from build123d import *

# Parameters (mm, degrees)
RESSALTO_EXTRUS_O1_DEPTH   = 5
CORTE_EXTRUS_O1_DEPTH      = 83.83115356
CORTE_EXTRUS_O1_DEPTH_BACK = 4
ESBO_O5_W                  = 35
ESBO_O5_H                  = 10
RESSALTO_EXTRUS_O2_DEPTH   = 5
FILETE1_R                  = 5
CORTE_EXTRUS_O2_DEPTH      = 83.83115356
CORTE_EXTRUS_O3_DEPTH      = 5
FILETE2_R                  = 2
ESBO_O10_W                 = 20
ESBO_O10_H                 = 50
CORTE_EXTRUS_O4_DEPTH      = 84.282651255


with BuildPart() as part:
    # Esboço1 → Ressalto-extrusão1 (new body)
    with BuildSketch(Plane.XY):
        Polygon((0, 0), (0, 70), (20, 70), (20, 20), (44, 20), (44, 0), align=None)
    extrude(amount=RESSALTO_EXTRUS_O1_DEPTH)

    # Esboço5 → Corte-extrusão1 (cut, two sides: drawn at the far end of the back side and taken through both)
    with BuildSketch(Plane.XY.offset(5).offset(-CORTE_EXTRUS_O1_DEPTH_BACK)):
        with Locations((26.5, 9)):
            Rectangle(ESBO_O5_W, ESBO_O5_H)
    extrude(amount=CORTE_EXTRUS_O1_DEPTH + CORTE_EXTRUS_O1_DEPTH_BACK, mode=Mode.SUBTRACT)

    # Esboço6 → Ressalto-extrusão2 (add)
    with BuildSketch(Plane.XY.offset(5)):
        Polygon((44, 20), (0, 20), (0, 0), (44, 0), (44, 4), (9, 4), (9, 14), (44, 14), align=None)
    extrude(amount=RESSALTO_EXTRUS_O2_DEPTH)

    # Filete1
    filete1_edges = [part.edges().sort_by_distance(p)[0] for p in [
        (10, 20, 5),
    ]]
    fillet(filete1_edges, radius=FILETE1_R - 0.0001)  # a hair under: the kernel refuses the full size

    # Esboço7 → Corte-extrusão2 (cut, through all)
    with BuildSketch(Plane.XY.offset(5)):
        with BuildLine():
            Line((12.75, 65), (12.75, 55))
            ThreePointArc((12.75, 55), (10, 52.25), (7.25, 55))
            Line((7.25, 55), (7.25, 65))
            ThreePointArc((7.25, 65), (10, 67.75), (12.75, 65))
        make_face()
    extrude(amount=-CORTE_EXTRUS_O2_DEPTH, mode=Mode.SUBTRACT)

    # Esboço8 → Corte-extrusão3 (cut)
    with BuildSketch(Plane.XZ):
        with BuildLine():
            Line((11.75, 8), (19.75, 8))
            ThreePointArc((19.75, 8), (22.5, 5.25), (19.75, 2.5))
            Line((19.75, 2.5), (11.75, 2.5))
            ThreePointArc((11.75, 2.5), (9, 5.25), (11.75, 8))
        make_face()
    extrude(amount=-CORTE_EXTRUS_O3_DEPTH, mode=Mode.SUBTRACT)

    # Filete2
    filete2_edges = [part.edges().sort_by_distance(p)[0] for p in [
        (0, 70, 2.5),
        (20, 70, 2.5),
    ]]
    fillet(filete2_edges, radius=FILETE2_R)

    # Esboço10 → Corte-extrusão4 (cut, through all)
    with BuildSketch(Plane.XY.offset(10)):
        with Locations((10, 45)):
            Rectangle(ESBO_O10_W, ESBO_O10_H)
    extrude(amount=-CORTE_EXTRUS_O4_DEPTH, mode=Mode.SUBTRACT)


solid = part.part
Source: CAD feature listing. Evaluate the final solid. Frame: model axes, mm. A direction names the side the tool comes from. Give positions to 0.01 mm unless a question says otherwise; leave off trailing zeros. Write each loop counter-clockwise with the first axis right and the second up, starting at its lowest first coordinate (ties: lowest second). Pieces come first, ordered by that corner, then holes. Notation, with made-up numbers: M 68,25.5 L 126,25.5 A22 ccw 126,56.5 Z; hole C 33.5,33 d10. An arc over 180 degrees is marked long. Return JSON: item names as keys, results as strings. Group by question number.
1) First-contact query: pin 1 Ø1 at (x, z) = (20, 4) entering from -Y; pin 2 Ø4.5 at (y, z) = (10.5, 3.5) entering from +X. Flat tips, straight axial feed; report the tip coordinate or a pass-through.
2) Cut plane B-B, the plane y = 1.5. Output: boundary loops of the cut face in (x, z).
3) Set-up query: faces 5 (the face through (9, 2, 5.2)), 6 (the face through (17, 15, 10)), 7 (the face through (31, 4, 5)). Return all of +Z, -Z, +X, -X, +Y, -Y with unobstructed straight access to the full face (end or side cutting, diameter ignored); none if empty.
4) Cut plane D-D, the plane y = 11.75. Output: boundary loops of the cut face in (x, z).
5) Draft query along X for faces 1 (the face through (0, 10, 5)), 2 (the face through (16, 2, 8)), 3 (the face through (22.5, 2, 5.3)), 4 (the face through (26, 9, 1)). Return one class per face: released by +X, released by -X, zero draft, split by the parting line, or undercut.
6) Cut plane A-A, the plane x = 17. Output: boundary loops of the cut face in (y, z), then the cut area to 3 significant figures.
7) Ray query, L1, parallel to Y at x = 31.5, z = 1.5; L2, parallel to Z at x = 25, y = 7; L3, parallel to X at y = 12.75, z = 5.75. Return the intervals inside material, ascending.
8) Cut plane C-C, the plane x = 25. Output: boundary loops of the cut face in (y, z), then the cut area to 3 significant figures.
Data:
{
 "1": {"pin 1": "stops at y = 14", "pin 2": "stops at x = 9"},
 "2": {"outline": "M 0,0 L 44,0 L 44,10 L 0,10 Z; hole M 11.75,2.5 L 19.75,2.5 A2.75 ccw 19.75,8 L 11.75,8 A2.75 ccw Z"},
 "3": {"face 5": "-Y", "face 6": "+Z, +X, -X, +Y, -Y", "face 7": "+Z, +X"},
 "4": {"outline": "M 0,0 L 44,0 L 44,1 L 9,1 L 9,10 L 0,10 Z"},
 "5": {"face 1": "released by -X", "face 2": "undercut", "face 3": "undercut", "face 4": "zero draft"},
 "6": {"outline": "M 0,0 L 20,0 L 20,10 L 14,10 L 14,1 L 4,1 L 4,2.5 L 0,2.5 Z; M 0,8 L 4,8 L 4,10 L 0,10 Z", "area": "88.0 mm²"},
 "7": {"L1": "y = 0 to 4, 14 to 20", "L2": "z = 0 to 1", "L3": "x = 0 to 9"},
 "8": {"outline": "M 0,0 L 20,0 L 20,10 L 14,10 L 14,1 L 4,1 L 4,10 L 0,10 Z", "area": "110 mm²"}
}
